from build123d import *

# Parameters (mm, degrees)
BOSS_EXTRUDE1_DEPTH = 4
BOSS_EXTRUDE1_DRAFT = 1
SHELL1_T            = -0.5
SKETCH2_R           = 2
BOSS_EXTRUDE2_DEPTH = 5.5
BOSS_EXTRUDE2_TAPER = 1.5
CIRPATTERN1_COUNT   = 4


with BuildPart() as part:
    # Sketch1 → Boss-Extrude1 (with draft: the straight prism first)
    with BuildSketch(Plane(origin=(0, 0, 0), x_dir=(1, 0, 0), z_dir=(0, 1, 0))):
        with BuildLine():
            Line((-7.5, -6.375), (7.5, -6.375))
            ThreePointArc((7.5, -6.375), (8.207106781, -6.082106781), (8.5, -5.375))
            Line((8.5, -5.375), (8.5, 5.375))
            ThreePointArc((8.5, 5.375), (8.207106781, 6.082106781), (7.5, 6.375))
            Line((7.5, 6.375), (-7.5, 6.375))
            ThreePointArc((-7.5, 6.375), (-8.207106781, 6.082106781), (-8.5, 5.375))
            Line((-8.5, 5.375), (-8.5, -5.375))
            ThreePointArc((-8.5, -5.375), (-8.207106781, -6.082106781), (-7.5, -6.375))
        make_face()
    extrude(amount=-BOSS_EXTRUDE1_DEPTH)
    # Boss-Extrude1: the draft: its side faces are tilted about the plane it starts from
    boss_extrude1_sides = [part.faces().sort_by_distance(p)[0] for p in [
        (0, -2, 6.375),
        (8.207106781, -2, 6.082106781),
        (8.5, -2, 0),
        (8.207106781, -2, -6.082106781),
        (0, -2, -6.375),
        (-8.207106781, -2, -6.082106781),
        (-8.5, -2, 0),
        (-8.207106781, -2, 6.082106781),
    ]]
    draft(boss_extrude1_sides, Plane(origin=(0, 0, 0), x_dir=(1, 0, 0), z_dir=(0, 1, 0)), BOSS_EXTRUDE1_DRAFT)

    # Shell1
    shell1_openings = [part.faces().sort_by_distance(p)[0] for p in [
        (0, -4, 0),
    ]]
    offset(amount=SHELL1_T, openings=shell1_openings, kind=Kind.INTERSECTION)

    # Sketch2 → Boss-Extrude2 (add)
    with BuildSketch(Plane.XZ.offset(0.5)):
        Circle(SKETCH2_R)
    extrude(amount=BOSS_EXTRUDE2_DEPTH, taper=BOSS_EXTRUDE2_TAPER)

    # Rib1: read off the stored shape, not the designer's step
    # Rib1: loft between two sections, ruled curve by curve
    rib1_from = [
        Edge.make_line((1.982020638, -0.5, 0.267570907), (3, -0.5, 0.25)),
        Edge.make_line((1.982020638, -0.5, -0.267570907), (3, -0.5, -0.25)),
        Edge.make_line((3, -0.5, -0.25), (3, -0.5, 0.25)),
        Edge.make_line((1.982020638, -0.5, -0.267570907), (1.982020638, -0.5, 0.267570907)),
    ]
    rib1_to = [
        Edge.make_line((1.87747837, -4.5, 0.258981593), (2.397831467, -4.5, 0.25)),
        Edge.make_line((1.87747837, -4.5, -0.258981593), (2.397831467, -4.5, -0.25)),
        Edge.make_line((2.397831467, -4.5, -0.25), (2.397831467, -4.5, 0.25)),
        Edge.make_line((1.87747837, -4.5, -0.258981593), (1.87747837, -4.5, 0.258981593)),
    ]
    rib1 = Solid(Shell([*[Face.make_surface_from_curves(rib1_from[k], rib1_to[k]) for k in range(4)], Face(Wire(rib1_from)), Face(Wire(rib1_to))]))
    add(rib1)

    # CirPattern1: Rib1 ×4 about axis
    cirpattern1_axis = Axis((0, 0, 0), (0, 1, 0))
    for i in range(1, CIRPATTERN1_COUNT):
        add(rib1.rotate(cirpattern1_axis, i * 360 / CIRPATTERN1_COUNT))


solid = part.part
Design review of the part built by this model. Coordinates are the model's own, in mm. A direction names the side the tool comes from. Coordinates: 2 decimals unless noted, no trailing zeros. Write each loop counter-clockwise with the first axis right and the second up, starting at its lowest first coordinate (ties: lowest second). Pieces come first, ordered by that corner, then holes. Notation, with made-up numbers: (-31.5, 74.5) - (6.5, 74.5) arc R24 ccw to (6.5, 108.5) - close; hole circle Ø9 at (56, 41). An arc over 180 degrees is marked (long way). Use one line per item in the form item = value.
Q1. For probe 1 along X at (y, z) = (-3.75, -4.25); probe 2 along Z at (x, y) = (4.75, -3.75); probe 3 along Z at (x, y) = (-2.25, -1.75), list the stretches that pass through material, from the lowest coordinate up.
Taken from the geometry:
probe_1 = -8.57 to -8.07, 8.07 to 8.57
probe_2 = -6.44 to -5.94, 5.94 to 6.44
probe_3 = -6.41 to -5.91, -0.26 to 0.26, 5.91 to 6.41
Q2. Consider section A-A (x = 3.75). Write out the cut boundary in (y, z) (3 decimals).
Taken from the geometry:
outline = (-4, -6.445) - (0, -6.375) - (0, 6.375) - (-4, 6.445) - (-4, 5.945) - (-0.5, 5.884) - (-0.5, -5.884) - (-4, -5.945) - close
Q3. Insertion check: pin 1 Ø3 at (y, z) = (-2, 2) entering from -X; pin 2 Ø5 at (x, z) = (-4.5, -3.5) entering from -Y; pin 3 Ø1 at (x, z) = (5, -5) entering from -Y. Each pin has a flat end and moves straight along its axis. Give the tip position at first contact, or say it passes through.
Taken from the geometry:
pin_1 = -8.56
pin_2 = -4
pin_3 = -0.5
Q4. Consider section C-C (y = -4.75). Write out the cut boundary in (x, z).
Taken from the geometry:
outline = circle Ø3.78 at (0, 0)
Q5. Machinability: for faces 1 (the flat face through (-2, -0.5, 1)), 2 (the conical face through (-8.223, -1.972, -6.114)), 3 (the conical face through (-8.24, -1.97, 6.1)), which of the approach directions +Z, -Z, +X, -X, +Y, -Y give a long, thin tool a straight path to every point of the face, cutting with its end or side? Answer none if there is none.
Taken from the geometry:
face_1 = -Y
face_2 = -Z, -X, +Y
face_3 = +Z, -X, +Y
Q6. The part is to be moulded in two halves that separate along Z. For faces 4 (the flat face through (0, -6, 0)), 5 (the conical face through (8.223, -1.972, 6.114)), 6 (the conical face through (8.24, -1.97, -6.1)), 7 (the conical face through (0.89, -3.29, -1.71)), say which applies: +Z half, -Z half, draft (parallel to the pull), parting line (faces both ways), or undercut.
Taken from the geometry:
face_4 = draft
face_5 = +Z half
face_6 = -Z half
face_7 = undercut
Q7. Consider section B-B (y = -0.75). Count the separate pieces of the cut face and the enclosed holes in it, plus the area to 3 significant figures.
Taken from the geometry:
separate_pieces = 2
enclosed_holes = 1
area = 42.7 mm^2
